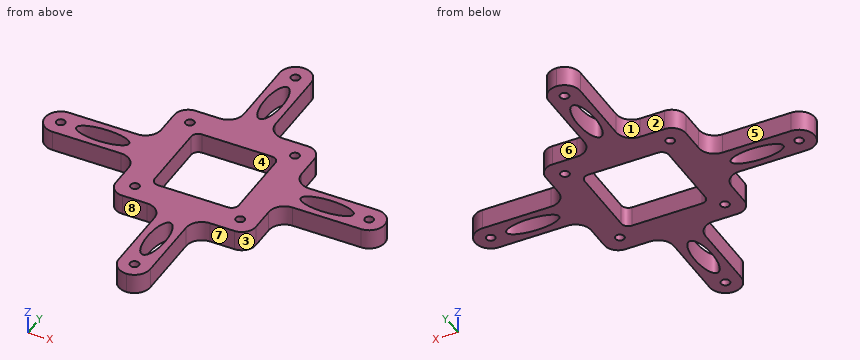
from build123d import *

# Parameters (mm, degrees)
SKETCH1_R           = 1.25
SKETCH1_RX          = 7.495001668
SKETCH1_RY          = 2.505000234
BOSS_EXTRUDE1_DEPTH = 5.8


with BuildPart() as part:
    # Sketch1 → Boss-Extrude1 (new body)
    with BuildSketch(Plane.XY):
        with BuildLine():
            Line((-16, 20), (-8.99, 20))
            ThreePointArc((-8.99, 20), (-5.815090552, 21.315090552), (-4.5, 24.49))
            Line((-4.5, 24.49), (-4.5, 44))
            ThreePointArc((-4.5, 44), (-3.181980515, 47.181980515), (0, 48.5))
            ThreePointArc((0, 48.5), (3.181980515, 47.181980515), (4.5, 44))
            Line((4.5, 44), (4.5, 24.49))
            ThreePointArc((4.5, 24.49), (5.815090552, 21.315090552), (8.99, 20))
            Line((8.99, 20), (16, 20))
            ThreePointArc((16, 20), (18.828427125, 18.828427125), (20, 16))
            Line((20, 16), (20, 8.99))
            ThreePointArc((20, 8.99), (21.315090552, 5.815090552), (24.49, 4.5))
            Line((24.49, 4.5), (44, 4.5))
            ThreePointArc((44, 4.5), (47.181980515, 3.181980515), (48.5, 0))
            ThreePointArc((48.5, 0), (47.181980515, -3.181980515), (44, -4.5))
            Line((44, -4.5), (24.49, -4.5))
            ThreePointArc((24.49, -4.5), (21.315090552, -5.815090552), (20, -8.99))
            Line((20, -8.99), (20, -16))
            ThreePointArc((20, -16), (18.828427125, -18.828427125), (16, -20))
            Line((16, -20), (8.99, -20))
            ThreePointArc((8.99, -20), (5.815090552, -21.315090552), (4.5, -24.49))
            Line((4.5, -24.49), (4.5, -44))
            ThreePointArc((4.5, -44), (3.181980515, -47.181980515), (0, -48.5))
            ThreePointArc((0, -48.5), (-3.181980515, -47.181980515), (-4.5, -44))
            Line((-4.5, -44), (-4.5, -24.49))
            ThreePointArc((-4.5, -24.49), (-5.815090552, -21.315090552), (-8.99, -20))
            Line((-8.99, -20), (-16, -20))
            ThreePointArc((-16, -20), (-18.828427125, -18.828427125), (-20, -16))
            Line((-20, -16), (-20, -8.99))
            ThreePointArc((-20, -8.99), (-21.315090552, -5.815090552), (-24.49, -4.5))
            Line((-24.49, -4.5), (-44, -4.5))
            ThreePointArc((-44, -4.5), (-47.181980515, -3.181980515), (-48.5, 0))
            ThreePointArc((-48.5, 0), (-47.181980515, 3.181980515), (-44, 4.5))
            Line((-44, 4.5), (-24.49, 4.5))
            ThreePointArc((-24.49, 4.5), (-21.315090552, 5.815090552), (-20, 8.99))
            Line((-20, 8.99), (-20, 16))
            ThreePointArc((-20, 16), (-18.828427125, 18.828427125), (-16, 20))
        make_face()
        with Locations((0, 44)):
            Circle(SKETCH1_R, mode=Mode.SUBTRACT)
        with Locations((-15, 15)):
            Circle(SKETCH1_R, mode=Mode.SUBTRACT)
        with Locations(Location((15, 15, 0), (0, 0, 180))):
            Circle(SKETCH1_R, mode=Mode.SUBTRACT)
        with Locations((15, -15)):
            Circle(SKETCH1_R, mode=Mode.SUBTRACT)
        with Locations(Location((-15, -15, 0), (0, 0, 180))):
            Circle(SKETCH1_R, mode=Mode.SUBTRACT)
        with Locations(Location((44, 0, 0), (0, 0, 180))):
            Circle(SKETCH1_R, mode=Mode.SUBTRACT)
        with Locations(Location((0, -44, 0), (0, 0, 180))):
            Circle(SKETCH1_R, mode=Mode.SUBTRACT)
        with Locations((-44, 0)):
            Circle(SKETCH1_R, mode=Mode.SUBTRACT)
        with Locations(Location((-0.004999676, 32.005), (0, 0, 89.961779812))):
            Ellipse(SKETCH1_RX, SKETCH1_RY, mode=Mode.SUBTRACT)
        with Locations(Location((32.005, -0.004999676), (0, 0, 0.038220188))):
            Ellipse(SKETCH1_RX, SKETCH1_RY, mode=Mode.SUBTRACT)
        with Locations(Location((-0.004999676, -32.005), (0, 0, -89.961779812))):
            Ellipse(SKETCH1_RX, SKETCH1_RY, mode=Mode.SUBTRACT)
        with Locations(Location((-32.005, -0.004999676), (0, 0, 179.961779812))):
            Ellipse(SKETCH1_RX, SKETCH1_RY, mode=Mode.SUBTRACT)
        with BuildLine():
            Line((9.99479618, -11.99479618), (-9.99479618, -11.99479618))
            ThreePointArc((-9.99479618, -11.99479618), (-11.409009742, -11.409009742), (-11.99479618, -9.99479618))
            Line((-11.99479618, -9.99479618), (-11.99479618, 9.99479618))
            ThreePointArc((-11.99479618, 9.99479618), (-11.409009742, 11.409009742), (-9.99479618, 11.99479618))
            Line((-9.99479618, 11.99479618), (9.99479618, 11.99479618))
            ThreePointArc((9.99479618, 11.99479618), (11.409009742, 11.409009742), (11.99479618, 9.99479618))
            Line((11.99479618, 9.99479618), (11.99479618, -9.99479618))
            ThreePointArc((11.99479618, -9.99479618), (11.409009742, -11.409009742), (9.99479618, -11.99479618))
        make_face(mode=Mode.SUBTRACT)
    extrude(amount=BOSS_EXTRUDE1_DEPTH)


solid = part.part
For this review, take the finished solid that the model builds, in its own axes (mm). Face numbers are marked on the shaded views. A direction names the side the tool comes from. Round coordinates to 2 decimals unless told otherwise and drop trailing zeros. Write each loop counter-clockwise with the first axis right and the second up, starting at its lowest first coordinate (ties: lowest second). Pieces come first, ordered by that corner, then holes. Notation, with made-up numbers: (58.5, 21) - (80.5, 21) arc R28 cw to (80.5, 54) - close; hole circle Ø7 at (-15.75, 33.25). An arc over 180 degrees is marked (long way). Write item = value, one per line. Start each with the question number.
1. For pin 1 Ø1.5 at (y, z) = (-1, 4.5) entering from +X; pin 2 Ø2 at (x, y) = (0, 44) entering from -Z; pin 3 Ø3 at (y, z) = (4, 1.5) entering from +X; pin 4 Ø1.7 at (x, z) = (32.5, 3.5) entering from +Y, all flat-tipped, find the tip position at first contact; note any pin that passes through.
2. Consider section A-A on y = -6. State the section outline as (x, z) points, plus the area to 3 significant figures.
3. Consider section B-B on z = 2.3. Give the number of separate pieces and of enclosed holes in the cut face, plus the area to 3 significant figures.
4. Wall thickness on L1, parallel to Y at x = -15, z = 1.4; L2, parallel to X at y = -32.5, z = 0.95; L3, parallel to X at y = -44, z = 2.4: over which ranges is each line inside the solid? List them lowest first.
5. For the marked faces 5, 6, 7 and 8, list the 3-axis set-ups (+Z, -Z, +X, -X, +Y, -Y) from which the entire face can be reached by the end or side of a thin tool; tool diameter is ignored.
6. Consider section C-C on y = 22. State the section outline as (x, z) points.
7. Draft analysis for pull direction X (two halves, no side actions). For the marked faces 1, 2, 3 and 4, state which applies: released by +X, released by -X, zero draft, split by the parting line, or undercut.
Evaluation:
q1.pin_1 = 48.49
q1.pin_2 = through
q1.pin_3 = 47.74
q1.pin_4 = 4.5
q2.outline = (-21.14, 0) - (-11.99, 0) - (-11.99, 5.8) - (-21.14, 5.8) - close; (11.99, 0) - (21.14, 0) - (21.14, 5.8) - (11.99, 5.8) - close
q2.area = 106 mm2
q3.separate_pieces = 1
q3.enclosed_holes = 13
q3.area = 1,760 mm2
q4.L1 = -20 to -16.25, -13.75 to 13.75, 16.25 to 20
q4.L2 = -4.5 to -2.5, 2.49 to 4.5
q4.L3 = -4.5 to -1.25, 1.25 to 4.5
q5.face_5 = +Z, -Z, -X, +Y
q5.face_6 = +Z, -Z, +X, +Y
q5.face_7 = +Z, -Z, +X, -Y
q5.face_8 = +Z, -Z, -X, -Y
q6.outline = (-5.25, 0) - (5.25, 0) - (5.25, 5.8) - (-5.25, 5.8) - close
q7.face_1 = released by -X
q7.face_2 = zero draft
q7.face_3 = released by +X
q7.face_4 = undercut
